from build123d import *

# Parameters (mm, degrees)
SKETCH1_W                    = 842
SKETCH1_H                    = 50
BOSS_EXTRUDE1_DEPTH          = 18
SKETCH2_W                    = 18
SKETCH2_H                    = 234.314907891
CUT_EXTRUDE1_DEPTH           = 5
F_4_0_4_DIAMETER_HOLE1_D     = 4
F_4_0_4_DIAMETER_HOLE1_DEPTH = 30
F_4_0_4_DIAMETER_HOLE1_TIP   = 1.201721238
F_4_0_4_DIAMETER_HOLE2_D     = 4
F_4_0_4_DIAMETER_HOLE2_DEPTH = 30
F_4_0_4_DIAMETER_HOLE2_TIP   = 1.201721238


with BuildPart() as part:
    # Sketch1 → Boss-Extrude1 (new body)
    with BuildSketch(Plane(origin=(0, 0, 0), x_dir=(1, 0, 0), z_dir=(0, 1, 0))):
        Rectangle(SKETCH1_W, SKETCH1_H)
    extrude(amount=BOSS_EXTRUDE1_DEPTH)

    # Sketch2 → Cut-Extrude1 (cut)
    with BuildSketch(Plane(origin=(0, 18, 0), x_dir=(1, 0, 0), z_dir=(0, 1, 0))):
        with Locations((-327, 12.382649644)):
            Rectangle(SKETCH2_W, SKETCH2_H)
        with Locations((-109, 12.382649644)):
            Rectangle(SKETCH2_W, SKETCH2_H)
        with Locations((109, 12.382649644)):
            Rectangle(SKETCH2_W, SKETCH2_H)
        with Locations((327, 12.382649644)):
            Rectangle(SKETCH2_W, SKETCH2_H)
    extrude(amount=-CUT_EXTRUDE1_DEPTH, mode=Mode.SUBTRACT)

    # Ø4.0 (4) Diameter Hole1
    with Locations(Plane.XY.offset(25)):
        with Locations((-320, 9), (-160, 9), (0, 9), (160, 9), (320, 9)):
            Hole(F_4_0_4_DIAMETER_HOLE1_D / 2, depth=F_4_0_4_DIAMETER_HOLE1_DEPTH)
            with Locations((0, 0, -(F_4_0_4_DIAMETER_HOLE1_DEPTH + F_4_0_4_DIAMETER_HOLE1_TIP / 2))):  # 118° drill point
                Cone(0, F_4_0_4_DIAMETER_HOLE1_D / 2, F_4_0_4_DIAMETER_HOLE1_TIP, mode=Mode.SUBTRACT)

    # Ø4.0 (4) Diameter Hole2
    with Locations(Plane(origin=(0, 0, -25), x_dir=(-1, 0, 0), z_dir=(0, 0, -1))):
        with Locations((-362.5, 9), (-217.5, 9), (-72.5, 9), (72.5, 9), (217.5, 9), (362.5, 9)):
            Hole(F_4_0_4_DIAMETER_HOLE2_D / 2, depth=F_4_0_4_DIAMETER_HOLE2_DEPTH)
            with Locations((0, 0, -(F_4_0_4_DIAMETER_HOLE2_DEPTH + F_4_0_4_DIAMETER_HOLE2_TIP / 2))):  # 118° drill point
                Cone(0, F_4_0_4_DIAMETER_HOLE2_D / 2, F_4_0_4_DIAMETER_HOLE2_TIP, mode=Mode.SUBTRACT)


solid = part.part
The model under review builds one solid part; all positions refer to its coordinate system, in mm. A direction names the side the tool comes from. Round coordinates to 2 decimals unless told otherwise and drop trailing zeros. Use a Markdown table: item, result. Add a question column.
Q1. The part is to be moulded in two halves that separate along X. For faces 3 (the face through (-421, 9, 0)), 4 (the face through (-1, 18, 0)), 5 (the face through (327, 13, 0)), say which applies: pulls with the +X half, pulls with the -X half, needs draft (parallel to the pull), parting line crosses it, or undercut.
Q2. Machinability: for faces 1 (the face through (-6, 9, -25)), 2 (the face through (-327, 13, 0)), which of the approach directions +Z, -Z, +X, -X, +Y, -Y give a long, thin tool a straight path to every point of the face, cutting with its end or side? Answer none if there is none.
Q3. Insertion check: pin 1 (5.5 mm diameter, centred on x = 107.5, z = 10, fed in from +Y); pin 2 (3 mm diameter, centred on x = 320, y = 9, fed in from +Z); pin 3 (3.5 mm diameter, centred on x = 72.5, y = 9, fed in from -Z). Each pin has a flat end and moves straight along its axis. Give the tip position at first contact, or say it passes through.
Q4. To check wall thickness, follow line 1 (X direction, y = 9.5, z = 19.5); line 2 (Y direction, x = 217, z = -4); line 3 (Y direction, x = 320, z = 9.5). State the ranges of each line that lie inside material, in increasing order.
Findings below:
| question | item | result |
|---|---|---|
| 1 | face 3 | pulls with the -X half |
| 1 | face 4 | needs draft |
| 1 | face 5 | undercut |
| 2 | face 1 | -Z, +X, -X, +Y, -Y |
| 2 | face 2 | +Z, -Z, +Y |
| 3 | pin 1 | stops at y = 13 |
| 3 | pin 2 | stops at z = -5.3 |
| 3 | pin 3 | stops at z = 5.15 |
| 4 | line 1 | x = -421 to -321.94, -318.06 to -161.94, -158.06 to -1.94, 1.94 to 158.06, 161.94 to 318.06, 321.94 to 421 |
| 4 | line 2 | y = 0 to 7.06, 10.94 to 18 |
| 4 | line 3 | y = 0 to 7, 11 to 13 |
